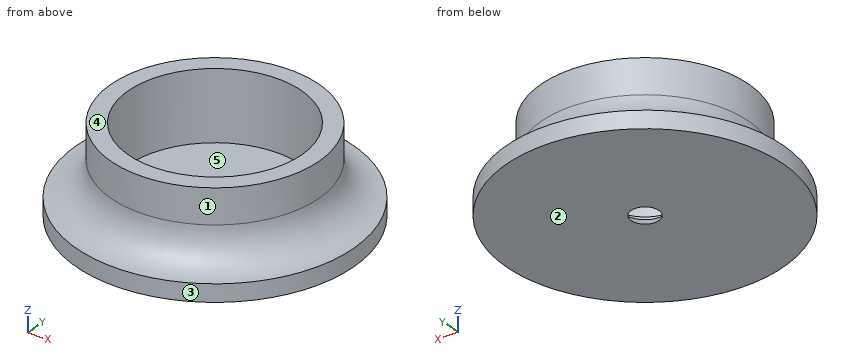
from build123d import *

# Parameters (mm, degrees)
CYLINDER_R         = 12.5
CYLINDER_DEPTH     = 10
CYLINDER001_R      = 15
CYLINDER001_DEPTH  = 10
TORUS_R            = 5
TUBE_R             = 20
TUBE_R_2           = 15
TUBE_DEPTH         = 5
CIRCLE002_R        = 4.6
EXTRUSION002_DEPTH = 1.3
CIRCLE001_R        = 2
EXTRUSION001_DEPTH = 42.073439
CIRCLE_R           = 20
EXTRUSION_DEPTH    = 2.5


with BuildPart() as cylinder:
    # Cylinder → Cylinder (new body)
    with BuildSketch(Plane.XY):
        Circle(CYLINDER_R)
    extrude(amount=CYLINDER_DEPTH)


with BuildPart() as cut:
    # Cylinder001 → Cylinder001 (new body)
    with BuildSketch(Plane.XY):
        Circle(CYLINDER001_R)
    extrude(amount=CYLINDER001_DEPTH)

    # Cut: cut Cylinder
    add(cylinder.part, mode=Mode.SUBTRACT)


with BuildPart() as torus:
    # Torus → Torus (revolve)
    with BuildSketch(Plane(origin=(0, 0, 5), x_dir=(1, 0, 0), z_dir=(0, -1, 0))):
        with Locations((20, 0)):
            Circle(TORUS_R)
    revolve(axis=Axis((0, 0, 5), (0, 0, 1)))


with BuildPart() as fusion:
    # Tube → Tube (new body)
    with BuildSketch(Plane.XY):
        Circle(TUBE_R)
        Circle(TUBE_R_2, mode=Mode.SUBTRACT)
    extrude(amount=TUBE_DEPTH)

    # Cut001: cut Torus
    add(torus.part, mode=Mode.SUBTRACT)

    # Fusion: union Cut
    add(cut.part)


with BuildPart() as cone:
    # Cone → Cone (revolve)
    with BuildSketch(Plane(origin=(0, 0, -2.5), x_dir=(1, 0, 0), z_dir=(0, -1, 0))):
        Polygon((0, 0), (2, 0), (3, 1.2), (0, 1.2), align=None)
    revolve(axis=Axis((0, 0, -2.5), (0, 0, 1)))


with BuildPart() as extrusion002:
    # Circle002 → Extrusion002 (new body)
    with BuildSketch(Plane.XY):
        Circle(CIRCLE002_R)
    extrude(amount=-EXTRUSION002_DEPTH)


with BuildPart() as extrusion001:
    # Circle001 → Extrusion001 (new body)
    with BuildSketch(Plane(origin=(0, 0, -2.5), x_dir=(1, 0, 0), z_dir=(0, 0, -1))):
        Circle(CIRCLE001_R)
    extrude(amount=-EXTRUSION001_DEPTH)


with BuildPart() as fusion001001:
    # Circle → Extrusion (new body)
    with BuildSketch(Plane(origin=(0, 0, 0), x_dir=(1, 0, 0), z_dir=(0, 0, -1))):
        Circle(CIRCLE_R)
    extrude(amount=EXTRUSION_DEPTH)

    # Cut002: cut Extrusion001
    add(extrusion001.part, mode=Mode.SUBTRACT)

    # Cut003: cut Extrusion002
    add(extrusion002.part, mode=Mode.SUBTRACT)

    # Cut004: cut Cone
    add(cone.part, mode=Mode.SUBTRACT)

    # Fusion001: union Fusion
    add(fusion.part)


with BuildPart() as fusion001001_1:
    # Fusion001001 placement: moved
    add(fusion001001.part.moved(Location((-49.230581, 0, 0))))


solid = fusion001001_1.part
Geometry check sheet. Reference: the model listing, model coordinates, mm. Face numbers are marked on the shaded views. A direction names the side the tool comes from. Give positions to 0.01 mm unless a question says otherwise; leave off trailing zeros. Order: outer loops, then holes, each group sorted by start corner. A loop starts at its lowest first (then second) coordinate and runs counter-clockwise, first axis right, second up. Notation, with made-up numbers: (82, 10) - (140, 10) arc R24 ccw to (140, 38) - close; hole circle Ø6 at (-23, 46). An arc over 180 degrees is marked (long way). Answer as a JSON object with one key per item and string values.
(1) Depth check by flat-ended pin: pin 1 Ø7.5 at (x, y) = (-49.23, 0) entering from +Z; pin 2 Ø1 at (x, z) = (-35, 5.5) entering from -Y; pin 3 Ø7.5 at (x, y) = (-43.5, 2.5) entering from +Z. Enter the tip coordinate at first touch or a pass-through.
Report:
{"pin 1": "z = -1.3", "pin 2": "y = -6.04", "pin 3": "z = 0"}
(2) Material ranges on line 1 (Z direction, x = -46, y = 7); line 2 (Y direction, x = -43, z = 0.5); line 3 (Y direction, x = -38, z = 9), recorded low to high.
Report:
{"line 1": "-2.5 to 0", "line 2": "-16.7 to -10.84, 10.84 to 16.7", "line 3": "-9.94 to -5.49, 5.49 to 9.94"}
(3) Tool access check on the marked faces 1 and 2. Record the directions out of +Z, -Z, +X, -X, +Y, -Y that give a thin tool (end or side, any length) a straight path to the whole face; none if there is none.
Report:
{"face 1": "+Z", "face 2": "-Z, +X, -X, +Y, -Y"}
(4) Draft check along Y on the marked faces 3, 4 and 5. Enter one of: released by +Y, released by -Y, zero draft, split by the parting line, or undercut.
Report:
{"face 3": "split by the parting line", "face 4": "zero draft", "face 5": "undercut"}
(5) Cross-section at A-A (z = 8.25). Record the cut outline in (x, y), then the cut area to 3 significant figures.
Report:
{"outline": "circle Ø30 at (-49.23, 0); hole circle Ø25 at (-49.23, 0)", "area": "216 mm^2"}
